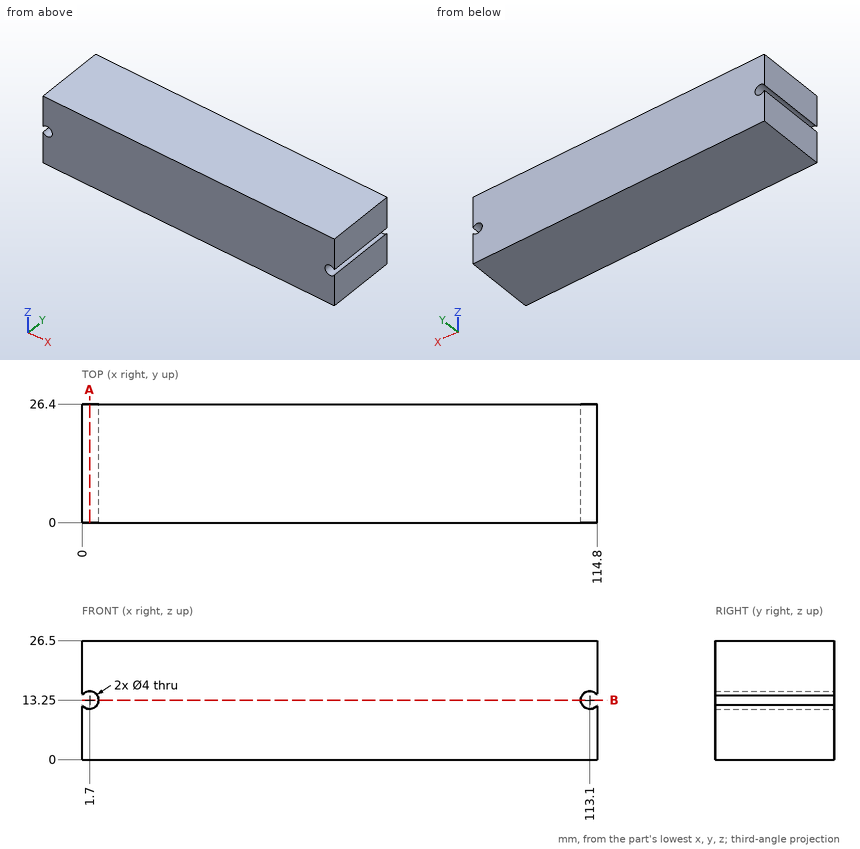
Geometry: see drawing. Coordinates: mm, zero at the bounding-box minimum. Coordinates: 2 decimals unless noted, no trailing zeros. Order: outer loops, then holes, each group sorted by start corner. A loop starts at its lowest first (then second) coordinate and runs counter-clockwise, first axis right, second up. Notation, with made-up numbers: (-11.5, -7.75) - (40.5, -7.75) arc R23 cw to (40.5, 4.25) - close; hole circle Ø4 at (72.5, 71.5). An arc over 180 degrees is marked (long way). Write each question's results on one line, items separated by ' | '.
1) Section B-B, the plane z = 13.25. Return loops of the section in (x, y), plus the area to 3 significant figures.
Results list:
outline: (3.7, 0) - (111.1, 0) - (111.1, 26.4) - (3.7, 26.4) - close | area: 2,840 mm^2
2) Section A-A, the plane x = 1.7. Return loops of the section in (y, z), plus the area to 3 significant figures.
Results list:
outline: (0, 0) - (26.4, 0) - (26.4, 11.25) - (0, 11.25) - close; (0, 15.25) - (26.4, 15.25) - (26.4, 26.5) - (0, 26.5) - close | area: 594 mm^2
3) Line query: line 1 (Z direction, x = 1.7, y = 15); line 2 (X direction, y = 8.25, z = 13.25). Output: solid intervals per line, ascending. Write a range as from..to.
Results list:
line 1: 0..11.25, 15.25..26.5 | line 2: 3.7..111.1
4) Pin query (flat end, axial travel): pin 1 (3 mm diameter, centred on x = 1.7, z = 13.25, fed in from +Y); pin 2 (5 mm diameter, centred on x = 90.5, y = 3.5, fed in from -Z). Return the tip coordinate at first contact, or that it passes through.
Results list:
pin 1: through | pin 2: z = 0
